Geometry: final body of the model. Coordinates: model frame, mm. Face numbers are marked on the shaded views. A direction names the side the tool comes from. Give positions to 0.01 mm unless a question says otherwise; leave off trailing zeros. Loops run counter-clockwise (first coordinate to the right, second up) from the corner with the lowest first, then second, coordinate; pieces in that order, holes last.
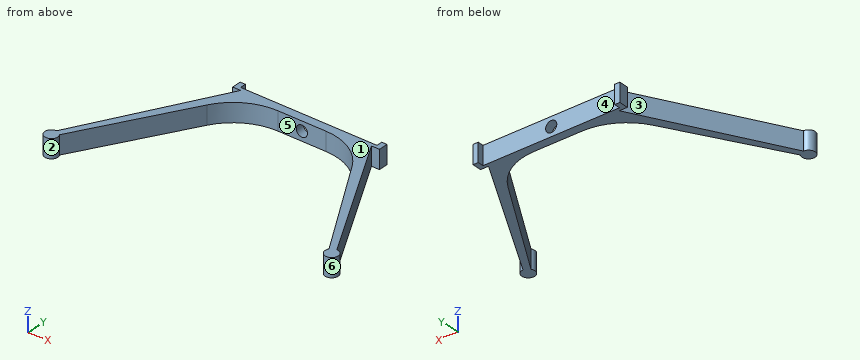
from build123d import *

# Parameters (mm, degrees)
F1_DEPTH = 10
F2_R     = 30
F3_W     = 78.57015
F3_H     = 10
F4_DEPTH = 5
F5_W     = 73.030218
F5_H     = 10
F6_DEPTH = 3.2
F7_R     = 3
F8_DEPTH = 7.801


with BuildPart() as f1:
    # F0 (on Top) → F1 (new body)
    with BuildSketch(Plane.XY):
        with BuildLine():
            Line((-35, 38.9), (-75, -34))
            ThreePointArc((-75, -34), (-76.683645, -40.568443), (-72.047904, -35.619806))
            Line((-72.047904, -35.619806), (-30.092474, 36.1))
            Line((-30.092474, 36.1), (30.092474, 36.1))
            Line((30.092474, 36.1), (72.047904, -35.619806))
            ThreePointArc((72.047904, -35.619806), (76.683645, -40.568443), (75, -34))
            Line((75, -34), (35, 38.9))
            Line((35, 38.9), (-35, 38.9))
        make_face()
    extrude(amount=F1_DEPTH)

    # F2
    f2_edges = [f1.edges().sort_by_distance(p)[0] for p in [
        (-30.092474, 36.1, 5),
        (30.092474, 36.1, 5),
    ]]
    fillet(f2_edges, radius=F2_R)

    # F3 (on face) → F4 (join)
    with BuildSketch(Plane(origin=(0, 38.9, 0), x_dir=(-1, 0, 0), z_dir=(0, 1, 0))):
        with Locations((0, 5)):
            Rectangle(F3_W, F3_H)
    extrude(amount=F4_DEPTH)

    # F5 (on face) → F6 (cut)
    with BuildSketch(Plane(origin=(0, 43.9, 0), x_dir=(-1, 0, 0), z_dir=(0, 1, 0))):
        with Locations((0, 5)):
            Rectangle(F5_W, F5_H)
    extrude(amount=-F6_DEPTH, mode=Mode.SUBTRACT)

    # F7 (on face) → F8 (cut, through all)
    with BuildSketch(Plane.XZ.offset(-36.1)):
        with Locations((0, 5)):
            Circle(F7_R)
    extrude(amount=-F8_DEPTH, mode=Mode.SUBTRACT)


solid = f1.part
Item 1: Draft query along X for the marked faces 1, 2 and 3. Return one class per face: +X half, -X half, draft (parallel to the pull), parting line (faces both ways), or undercut.
Values follow:
face 1: draft
face 2: undercut
face 3: -X half
Item 2: Ray query, probe 1 along Z at (x, y) = (0, 38); probe 2 along X at (y, z) = (-35.5, 7.75); probe 3 along X at (y, z) = (-36, 9.25). Return the intervals inside material, ascending.
Values follow:
probe 1: z = 0 to 2, 8 to 10
probe 2: x = -77.87 to -71.98, 71.98 to 77.87
probe 3: x = -78.16 to -71.84, 71.84 to 78.16
Item 3: Section query D-D on x = -19.5. Return loops of the section in (y, z), plus the area to 3 significant figures.
Values follow:
outline: (35.36, 0) - (40.7, 0) - (40.7, 10) - (35.36, 10) - close
area: 53.4 mm2
Item 4: Section query A-A on y = -37.5. Return loops of the section in (x, z).
Values follow:
outline: (-78.5, 0) - (-71.5, 0) - (-71.5, 10) - (-78.5, 10) - close; (71.5, 0) - (78.5, 0) - (78.5, 10) - (71.5, 10) - close
Item 5: Section query B-B on x = 0. Return loops of the section in (y, z), plus the area to 3 significant figures.
Values follow:
outline: (36.1, 0) - (40.7, 0) - (40.7, 2) - (36.1, 2) - close; (36.1, 8) - (40.7, 8) - (40.7, 10) - (36.1, 10) - close
area: 18.4 mm2
Item 6: Section query C-C on z = 5. Return loops of the section in (x, y), plus the area to 3 significant figures.
Values follow:
outline: (-75, -34) arc R3.5 ccw (long way) to (-72.05, -35.62) - (-38.78, 21.25) arc R30 cw to (-12.89, 36.1) - (-3, 36.1) - (-3, 40.7) - (-36.52, 40.7) - (-36.52, 43.9) - (-39.29, 43.9) - (-39.29, 38.9) - (-35, 38.9) - close; (3, 36.1) - (12.89, 36.1) arc R30 cw to (38.78, 21.25) - (72.05, -35.62) arc R3.5 ccw (long way) to (75, -34) - (35, 38.9) - (39.29, 38.9) - (39.29, 43.9) - (36.52, 43.9) - (36.52, 40.7) - (3, 40.7) - close
area: 1,230 mm2
Item 7: Pin query (flat end, axial travel): pin 1 (4 mm diameter, centred on x = 22.5, z = 1.5, fed in from -Y); pin 2 (5 mm diameter, centred on x = 5, z = 5, fed in from -Y); pin 3 (2.5 mm diameter, centred on y = 42, z = 7, fed in from -X); pin 4 (10 mm diameter, centred on x = -47.5, y = 21, fed in from +Z). Return the tip coordinate at first contact, or that it passes through.
Values follow:
pin 1: stops at y = 33.76
pin 2: stops at y = 36.1
pin 3: stops at x = -39.29
pin 4: stops at z = 10
Item 8: Set-up query: the marked faces 4, 5 and 6. Return all of +Z, -Z, +X, -X, +Y, -Y with unobstructed straight access to the full face (end or side cutting, diameter ignored); none if empty.
Values follow:
face 4: +Z, -Z, +Y
face 5: +Z, -Z, -Y
face 6: +Z, -Z
